Check sheet for the modelled part. Datum: model origin and axes. Units: mm. Round coordinates to 2 decimals unless told otherwise and drop trailing zeros. Write each loop counter-clockwise with the first axis right and the second up, starting at its lowest first coordinate (ties: lowest second). Pieces come first, ordered by that corner, then holes. Notation, with made-up numbers: M -18,70 L -13,70 A12 cw -13,78 Z; hole C 0.25,6.25 d2. An arc over 180 degrees is marked long. One line per item, written item: value.
Autodesk Inventor part; units mm, degrees
ref_plane "YZ Plane" through (0, 0, 0) normal (1, 0, 0) x (0, 1, 0)
ref_plane "XZ Plane" through (0, 0, 0) normal (0, 1, 0) x (-1, 0, 0)
ref_plane "XY Plane" through (0, 0, 0) normal (0, 0, 1) x (1, 0, 0)
sketch "Sketch1" plane through (0, 0, 0) normal (0, 1, 0) x (-1, 0, 0)
  line L0 (0, 0) -> (0, -189.323) construction
  line L1 (-3, 0) -> (-3, -189.323)
  line L2 (3, -189.323) -> (3, 0)
  arc A0 (3, 0) -> (-3, 0) centre (0, 0) ccw
  arc A1 (-3, -189.323) -> (3, -189.323) centre (0, -189.323) ccw
  circle A2 centre (0, 0) radius 1.5
  circle A3 centre (0, -189.323) radius 1.5
  circle A4 centre (0, -111.208) radius 1.5
  point P0 (0, -94.6615)
  dimension "d0" = 189.323
  dimension "d1" = 6
  dimension "d2" = 3
  dimension "d3" = 3
  dimension "d6" = 3
  dimension "d7" = 111.208
extrude "Extrusion1" add sketch "Sketch1" along normal blind 8
sketch "Sketch2" plane through (0, 0, 0) normal (0, -1, 0) x (1, 0, 0)
  arc A0 (-3, -189.323) -> (3, -189.323) centre (0, -189.323) ccw
  line L0 (3, 0) -> (3, -189.323)
  arc A1 (3, 0) -> (-3, 0) centre (0, 0) ccw
  line L1 (-3, -189.323) -> (-3, 0)
  circle A2 centre (0, -111.208) radius 1.5
  circle A3 centre (0, -189.323) radius 1.5
  circle A4 centre (0, 0) radius 1.5
Q1. Sectioned sample at A-A on x = 0. Enter the section's corners in (y, z), and give its area (3 significant figures).
Completed:
outline: M 0,-192.32 L 8,-192.32 L 8,-190.82 L 0,-190.82 Z; M 0,-187.82 L 8,-187.82 L 8,-112.71 L 0,-112.71 Z; M 0,-109.71 L 8,-109.71 L 8,-1.5 L 0,-1.5 Z; M 0,1.5 L 8,1.5 L 8,3 L 0,3 Z
area: 1,490 mm^2
Q2. Sectioned sample at B-B on y = 5.5. Enter the section's corners in (x, z), and give its area (3 significant figures).
Completed:
outline: M -3,-189.32 A3 ccw 3,-189.32 L 3,0 A3 ccw -3,0 Z; hole C 0,-189.32 d3; hole C 0,-111.21 d3; hole C 0,0 d3
area: 1,140 mm^2
Q3. Scan lines: line 1 (Z direction, x = 0, y = 4); line 2 (Z direction, x = -1.85, y = 2); line 3 (Z direction, x = 1.65, y = 3.5). Record each from-to range of solid material in increasing order. Write a range as [from, to].
Completed:
line 1: [-192.32, -190.82], [-187.82, -112.71], [-109.71, -1.5], [1.5, 3]
line 2: [-191.68, 2.36]
line 3: [-191.83, 2.51]
Q4. Draft check along Z on faces 1 (the flat face through (0, 8, -93)), 2 (the cylindrical face through (-0.066, 3.944, -192.322)), 3 (the cylindrical face through (1.5, 3.94, -0.07)). Enter one of: pulls with the +Z half, pulls with the -Z half, needs draft (parallel to the pull), parting line crosses it, or undercut.
Completed:
face 1: needs draft
face 2: pulls with the -Z half
face 3: undercut
Q5. Depth check by flat-ended pin: P1, Ø2.5, axis at x = 0, z = -111.208, coming from the -Y side. Enter the tip coordinate at first touch or a pass-through.
Completed:
P1: through
